Read the model definition and answer for the solid it produces. Units are mm, in the model's axes. Face numbers are marked on the shaded views. Coordinates: 2 decimals unless noted, no trailing zeros. Loops run counter-clockwise (first coordinate to the right, second up) from the corner with the lowest first, then second, coordinate; pieces in that order, holes last. Notation, with made-up numbers: (65.25, 19) -> (114.25, 19) arc R18 ccw to (114.25, 54) -> close; hole circle Ø11 at (51.25, 12.5). An arc over 180 degrees is marked (long way). Answer in a Markdown table with one row per item.
```python
from build123d import *

# Parameters (mm, degrees)
SKETCH1_R             = 85
BOSS_EXTRUDE1_DEPTH   = 20
SKETCH2_R             = 27.5
CUT_EXTRUDE1_DEPTH    = 122.86057607
SKETCH3_R             = 2.80475321
CUT_EXTRUDE2_DEPTH    = 17.664904
CIRPATTERN1_START     = 2.335095674
CIRPATTERN1_OUTLINE_R = 2.80475321
CIRPATTERN1_DEPTH     = 17.664904326


# Read off the part's stored shape, not the designer's step: CirPattern1
with BuildPart() as part:
    # Sketch1 → Boss-Extrude1 (new body)
    with BuildSketch(Plane(origin=(0, 0, 0), x_dir=(1, 0, 0), z_dir=(0, 1, 0))):
        with Locations(Location((0, 0, 0), (0, 0, 270))):
            Circle(SKETCH1_R)
    extrude(amount=BOSS_EXTRUDE1_DEPTH)

    # Sketch2 → Cut-Extrude1 (cut, through all)
    with BuildSketch(Plane(origin=(0, 0, 0), x_dir=(1, 0, 0), z_dir=(0, 1, 0))):
        with Locations(Location((0, 0, 0), (0, 0, 270))):
            Circle(SKETCH2_R)
    extrude(amount=CUT_EXTRUDE1_DEPTH, mode=Mode.SUBTRACT)

    # Sketch3 → Cut-Extrude2 (cut)
    with BuildSketch(Plane(origin=(0, 20, 0), x_dir=(1, 0, 0), z_dir=(0, 1, 0))):
        with Locations(Location((-37.09345141, 0, 0), (0, 0, 270))):
            Circle(SKETCH3_R)
    extrude(amount=-CUT_EXTRUDE2_DEPTH, mode=Mode.SUBTRACT)

    # CirPattern1 outline → CirPattern1 (cut)
    with BuildSketch(Plane(origin=(0, 0, 0), x_dir=(1, 0, 0), z_dir=(0, 1, 0)).offset(CIRPATTERN1_START)):
        with Locations((-11.462506866, 35.277968675)):
            Circle(CIRPATTERN1_OUTLINE_R)
        with Locations((30.009232571, 21.802983695)):
            Circle(CIRPATTERN1_OUTLINE_R)
        with Locations((30.009232571, -21.802983695)):
            Circle(CIRPATTERN1_OUTLINE_R)
        with Locations((-11.462506866, -35.277968675)):
            Circle(CIRPATTERN1_OUTLINE_R)
    extrude(amount=CIRPATTERN1_DEPTH, mode=Mode.SUBTRACT)


solid = part.part
```
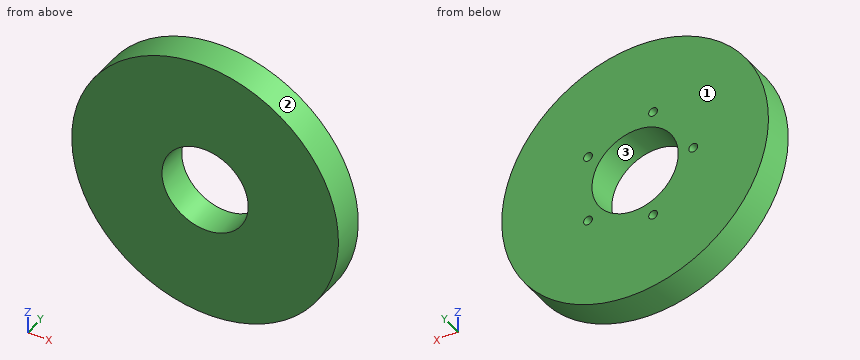
1. Find the intervals of material crossed by probe 1 along X at (y, z) = (5.5, 20); probe 2 along Z at (x, y) = (-18.5, 9.25); probe 3 along X at (y, z) = (8, 76), in increasing order.
A:
| item | result |
|---|---|
| probe 1 | x = -82.61 to -18.87, 18.87 to 27.86, 32.16 to 82.61 |
| probe 2 | z = -82.96 to -20.35, 20.35 to 82.96 |
| probe 3 | x = -38.07 to 38.07 |
2. A cutting plane is placed at B-B on x = 0. Give the vertices of the cut face in (y, z), and give its area (3 significant figures).
A:
| item | result |
|---|---|
| outline | (0, -85) -> (20, -85) -> (20, -27.5) -> (0, -27.5) -> close; (0, 27.5) -> (20, 27.5) -> (20, 85) -> (0, 85) -> close |
| area | 2,300 mm2 |
3. Given pin 1 Ø6 at (y, z) = (7, -47.5) entering from +X; pin 2 Ø1.5 at (x, y) = (40, 5) entering from -Z; pin 3 Ø1.5 at (x, y) = (-64, 7.5) entering from +Z, each flat-ended and moving along its own axis, determine where each tip first touches the part or whether it passes through.
A:
| item | result |
|---|---|
| pin 1 | stops at x = 72.42 |
| pin 2 | stops at z = -75.4 |
| pin 3 | stops at z = 56.78 |
4. A cutting plane is placed at D-D on x = -19.5. Give the vertices of the cut face in (y, z), and give its area (3 significant figures).
A:
| item | result |
|---|---|
| outline | (0, -82.73) -> (20, -82.73) -> (20, -19.39) -> (0, -19.39) -> close; (0, 19.39) -> (20, 19.39) -> (20, 82.73) -> (0, 82.73) -> close |
| area | 2,530 mm2 |
5. A cutting plane is placed at C-C on y = 5. Give the vertices of the cut face in (x, z), and give its area (3 significant figures).
A:
| item | result |
|---|---|
| outline | circle Ø170 at (0, 0); hole circle Ø5.61 at (-37.09, 0); hole circle Ø55 at (0, 0); hole circle Ø5.61 at (-11.46, -35.28); hole circle Ø5.61 at (-11.46, 35.28); hole circle Ø5.61 at (30.01, -21.8); hole circle Ø5.61 at (30.01, 21.8) |
| area | 20,200 mm2 |
6. A cutting plane is placed at A-A on z = 0. Give the vertices of the cut face in (x, y).
A:
| item | result |
|---|---|
| outline | (-85, 0) -> (-27.5, 0) -> (-27.5, 20) -> (-34.29, 20) -> (-34.29, 2.34) -> (-39.9, 2.34) -> (-39.9, 20) -> (-85, 20) -> close; (27.5, 0) -> (85, 0) -> (85, 20) -> (27.5, 20) -> close |
7. The mould has two halves that part along Z. Classify the marked faces 1, 2 and 3: pulls with the +Z half, pulls with the -Z half, needs draft (parallel to the pull), parting line crosses it, or undercut.
A:
| item | result |
|---|---|
| face 1 | needs draft |
| face 2 | parting line crosses it |
| face 3 | undercut |
